Autodesk Inventor part; units mm, degrees
ref_plane "YZ Plane" through (0, 0, 0) normal (1, 0, 0) x (0, 1, 0)
ref_plane "XZ Plane" through (0, 0, 0) normal (0, 1, 0) x (-1, 0, 0)
ref_plane "XY Plane" through (0, 0, 0) normal (0, 0, 1) x (1, 0, 0)
sketch "スケッチ1" plane through (0, 0, 0) normal (0, 0, 1) x (1, 0, 0)
  line L0 (-32.25, 65) -> (32.25, 65)
  line L1 (32.25, 65) -> (32.25, 47.1)
  line L2 (-32.25, -65) -> (-32.25, -47.1)
  line L3 (-32.25, 65) -> (32.25, -65) construction
  line L4 (32.25, 65) -> (-32.25, -65) construction
  line L5 (-32.25, 45) -> (-37.25, 45)
  line L6 (-37.25, 15) -> (-32.25, 15)
  line L7 (-37.25, 15) -> (-37.25, 45)
  line L8 (-32.25, -15) -> (-37.25, -15)
  line L9 (-37.25, -15) -> (-37.25, -45)
  line L10 (-37.25, -45) -> (-32.25, -45)
  arc A0 (-32.25, 45) -> (-32.25, 47.1) centre (-32.25, 46.05) ccw
  arc A1 (-32.25, 12.9) -> (-32.25, 15) centre (-32.25, 13.95) ccw
  arc A2 (-32.25, -15) -> (-32.25, -12.9) centre (-32.25, -13.95) ccw
  arc A3 (-32.25, -47.1) -> (-32.25, -45) centre (-32.25, -46.05) ccw
  line L11 (-32.25, 47.1) -> (-32.25, 65)
  line L12 (-32.25, 12.9) -> (-32.25, 15) construction
  line L13 (-32.25, -12.9) -> (-32.25, 12.9)
  line L14 (-32.25, -47.1) -> (-32.25, -45) construction
  line L15 (0, 65) -> (0, -65) construction
  arc A4 (32.25, -45) -> (32.25, -47.1) centre (32.25, -46.05) ccw
  line L16 (37.25, -45) -> (32.25, -45)
  line L17 (37.25, -15) -> (37.25, -45)
  line L18 (32.25, -15) -> (37.25, -15)
  arc A5 (32.25, -12.9) -> (32.25, -15) centre (32.25, -13.95) ccw
  arc A6 (32.25, 15) -> (32.25, 12.9) centre (32.25, 13.95) ccw
  line L19 (37.25, 15) -> (37.25, 45)
  line L20 (37.25, 15) -> (32.25, 15)
  line L21 (32.25, 45) -> (37.25, 45)
  arc A7 (32.25, 47.1) -> (32.25, 45) centre (32.25, 46.05) ccw
  line L22 (32.25, 47.1) -> (32.25, 45) construction
  line L23 (32.25, 12.9) -> (32.25, -12.9)
  line L24 (32.25, -47.1) -> (32.25, -65)
  line L25 (32.25, -12.9) -> (32.25, -15) construction
  line L26 (-32.25, -15) -> (-32.25, -12.9) construction
  line L27 (-32.25, -45) -> (-32.25, -15)
  line L28 (32.25, -15) -> (32.25, -45)
  line L29 (32.25, -45) -> (32.25, -47.1) construction
  line L30 (-20, -11.25) -> (-15, -11.25) construction
  line L31 (-15, -11.25) -> (-15, -31.25) construction
  line L32 (-15, -31.25) -> (-20, -31.25) construction
  line L33 (-20, -31.25) -> (-20, -11.25) construction
  line L34 (-20, -11.25) -> (-15, -31.25) construction
  line L35 (-15, -11.25) -> (-20, -31.25) construction
  line L36 (-20, 2.5) -> (-15, 2.5) construction
  line L37 (-15, 2.5) -> (-15, -45) construction
  line L38 (-15, -45) -> (-20, -45) construction
  line L39 (-20, -45) -> (-20, 2.5) construction
  line L40 (-20, 2.5) -> (-15, -45) construction
  line L41 (-15, 2.5) -> (-20, -45) construction
  circle A8 centre (-17.5, -36.25) radius 1.55
  line L42 (-20, -21.25) -> (-15, -21.25) construction
  line L43 (-17.5, 2.5) -> (-17.5, -45) construction
  circle A9 centre (-17.5, -6.25) radius 1.55
  circle A10 centre (17.5, -36.25) radius 1.55
  circle A11 centre (17.5, -6.25) radius 1.55
  line L44 (32.25, -65) -> (16.75, -65)
  line L45 (-12.5, -62.5) -> (-12.5, -45)
  line L46 (-12.5, -45) -> (0, -45)
  line L47 (12.5, -62.5) -> (12.5, -45)
  line L48 (12.5, -45) -> (0, -45)
  line L49 (-16.75, -65) -> (-32.25, -65)
  line L50 (16.75, -65) -> (-16.75, -65)
  line L51 (-32.25, 45) -> (-32.25, 47.1) construction
  line L52 (-32.25, 15) -> (-32.25, 45)
  line L53 (32.25, 15) -> (32.25, 12.9) construction
  line L54 (32.25, 45) -> (32.25, 15)
  circle A12 centre (-24.5, 43.5) radius 1.25
  line L55 (-32.25, 0) -> (32.25, 0) construction
  line L56 (-32.25, 46.5) -> (32.25, 46.5) construction
  circle A13 centre (-24.5, -61.5) radius 1.25
  circle A14 centre (24.5, 43.5) radius 1.25
  circle A15 centre (24.5, -61.5) radius 1.25
  circle A16 centre (-17.5, -36.25) radius 3 construction
  line L57 (-12.5, -62.5) -> (12.5, -62.5)
  line L58 (-24.25, 40.5) -> (24.25, 40.5)
  line L59 (24.25, 2.5) -> (-24.25, 2.5)
  line L60 (-24.25, 2.5) -> (-24.25, 40.5)
  line L61 (24.25, 2.5) -> (24.25, 40.5)
  line L62 (-20.05, -29.8151) -> (-18.5651, -31.3) construction
  line L63 (-19.3075, -30.5575) -> (-20.05, -31.3) construction
  arc A17 (-20.05, -29.8151) -> (-18.5651, -31.3) centre (-19.3075, -30.5575) ccw
  line L64 (-20.05, -11.2) -> (-18.5651, -11.2) construction
  line L65 (-14.95, -11.2) -> (-14.95, -12.6849) construction
  line L66 (-14.95, -31.3) -> (-16.4349, -31.3) construction
  line L67 (-20.05, -31.3) -> (-20.05, -29.8151) construction
  line L68 (-20.05, -11.2) -> (-14.95, -31.3) construction
  line L69 (-14.95, -11.2) -> (-20.05, -31.3) construction
  arc A18 (-16.4349, -31.3) -> (-14.95, -29.8151) centre (-15.6925, -30.5575) ccw
  arc A19 (-18.5651, -11.2) -> (-20.05, -12.6849) centre (-19.3075, -11.9425) ccw
  arc A20 (-14.95, -12.6849) -> (-16.4349, -11.2) centre (-15.6925, -11.9425) ccw
  line L70 (-20.05, -29.8151) -> (-20.05, -12.6849)
  line L71 (-18.5651, -31.3) -> (-20.05, -31.3) construction
  line L72 (-16.4349, -31.3) -> (-18.5651, -31.3)
  line L73 (-14.95, -29.8151) -> (-14.95, -31.3) construction
  line L74 (-20.05, -12.6849) -> (-20.05, -11.2) construction
  line L75 (-18.5651, -11.2) -> (-16.4349, -11.2)
  line L76 (-16.4349, -11.2) -> (-14.95, -11.2) construction
  line L77 (-14.95, -12.6849) -> (-14.95, -29.8151)
  arc A21 (18.5651, -31.3) -> (20.05, -29.8151) centre (19.3075, -30.5575) ccw
  arc A22 (14.95, -29.8151) -> (16.4349, -31.3) centre (15.6925, -30.5575) ccw
  arc A23 (16.4349, -11.2) -> (14.95, -12.6849) centre (15.6925, -11.9425) ccw
  arc A24 (20.05, -12.6849) -> (18.5651, -11.2) centre (19.3075, -11.9425) ccw
  line L78 (20.05, -29.8151) -> (20.05, -12.6849)
  line L79 (16.4349, -31.3) -> (18.5651, -31.3)
  line L80 (18.5651, -11.2) -> (16.4349, -11.2)
  line L81 (14.95, -12.6849) -> (14.95, -29.8151)
  line L82 (-32.25, -65) -> (-32.25, -70)
  line L83 (-32.25, -70) -> (32.25, -70)
  line L84 (32.25, -70) -> (32.25, -65)
  point P0 (0, 0)
  point P1 (0, 0)
  point P2 (0, 0)
  point P3 (28, 15)
  point P4 (28, 45)
  point P5 (-17.5, -21.25)
  point P6 (28, 45)
  point P7 (28, 15)
  dimension "d0" = 64.5
  dimension "d1" = 130
  dimension "d2" = 20
  dimension "d3" = 30
  dimension "d4" = 30
  dimension "d5" = 30
  dimension "d6" = 1.05
  dimension "d7" = 1.05
  dimension "d8" = 1.05
  dimension "d9" = 1.05
  dimension "d10" = 5
  dimension "d23" = 15
  dimension "d24" = 5
  dimension "d25" = 20
  dimension "d28" = 3.1
  dimension "d72" = 47.5
  dimension "d103" = 12.25
  dimension "d109" = 71.25
  dimension "d111" = 20
  dimension "d113" = 7.75
  dimension "d114" = 2.5
  dimension "d115" = 18.5
  dimension "d116" = 3
  dimension "d117" = 2.5
  dimension "d118" = 7.75
  dimension "d119" = 3.5
  dimension "d120" = 25
  dimension "d121" = 6
  dimension "d124" = 2.5
  dimension "d126" = 8
  dimension "d128" = 6
  dimension "d130" = 1.05
  dimension "d131" = 0.05
  dimension "d132" = 0.05
  dimension "d133" = 5
  dimension "d157" = 25
  dimension "d158" = 30
extrude "押し出し1" add sketch "スケッチ1" along normal blind 2.5 contours L0 L1 A7 L54 A6 L23 A5 L28 A4 L24 L44 L50 L49 L2 A3 L27 A2 L13 A1 L52 A0 L11 | L52 L6 L7 L5 | L21 L19 L20 L54 | L27 L10 L9 L8 | L18 L17 L16 L28
extrude "押し出し2" add sketch "スケッチ1" along normal blind 5 contours L0 L1 A7 L54 A6 L23 A5 L28 A4 L24 L44 L50 L49 L2 A3 L27 A2 L13 A1 L52 A0 L11
fillet "フィレット1" radius 1 7 edges at (-12.5, -45, 2.5) (-12.5, -62.5, 2.5) (12.5, -62.5, 2.5) (-24.25, 40.5, 2.5) (24.25, 40.5, 2.5) (24.25, 2.5, 2.5) (-24.25, 2.5, 2.5)
sketch "スケッチ7" plane through (32.25, -70, 0) normal (1, 0, 0) x (0, 0, -1)
  line L0 (0, 55) -> (-2.5, 55)
  line L1 (0, 57.1) -> (0, 82.9)
  line L2 (0, 5) -> (0, 22.9)
  point P0 (0, 70)
  point P1 (-2.5, 15)
  point P2 (-2.5, 65)
  point P3 (0, 25)
  dimension "d136" = 10
  dimension "d137" = 10
  dimension "d138" = 2.5
  dimension "d139" = 2.5
hole "穴6" at (32.25, -55, 2.5) at (32.25, -5, 2.5) direction (-1, 0, 0) diameter 2.459 depth 4
sketch "スケッチ8" plane through (-32.25, -70, 0) normal (-1, 0, 0) x (0, 0, 1)
  circle A0 centre (2.5, 15) radius 1.2295
  circle A1 centre (2.5, 65) radius 1.2295
  point P0 (0, 70)
  point P1 (2.5, 15)
  point P2 (2.5, 65)
hole "穴7" at (-32.25, -5, 2.5) at (-32.25, -55, 2.5) direction (1, 0, 0) diameter 2.459 depth 4
chamfer "面取り2" distance 0.5 angle 45 8 edges at (-37.25, -45, 1.25) (-37.25, -15, 1.25) (-37.25, 15, 1.25) (-37.25, 45, 1.25) (37.25, 15, 1.25) (37.25, 45, 1.25) (37.25, -15, 1.25) (37.25, -45, 1.25)
equation "\"d2\" = -0.5 * d4 + 0.5 * d1 - d3"
equation "\"d5\" = d3"
equation "\"d7\" = d6"
equation "\"d8\" = d7"
equation "\"d9\" = d8"
properties part number "Cockpit_upper_bottom_frame" material "アセタール樹脂、黒"
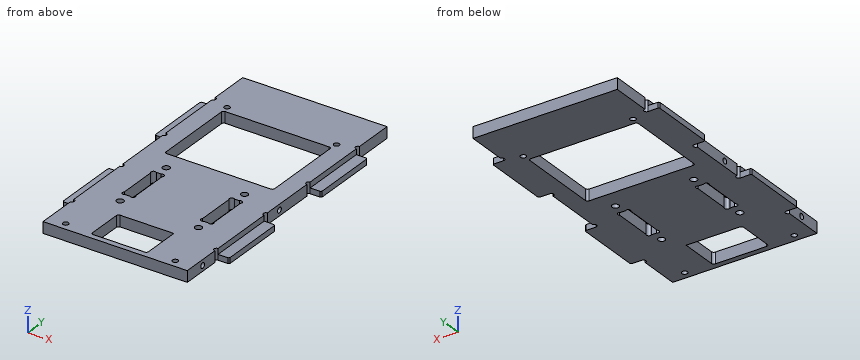
Work out the finished part from the listing and answer in its coordinate system (mm). Give positions to 0.01 mm unless a question says otherwise; leave off trailing zeros. Write each loop counter-clockwise with the first axis right and the second up, starting at its lowest first coordinate (ties: lowest second). Pieces come first, ordered by that corner, then holes. Notation, with made-up numbers: M 53,42 L 111,42 A27 ccw 111,71 Z; hole C 76.5,66 d9. An arc over 180 degrees is marked long. Answer as CSV lines item,"result".
Q1. A cutting plane is placed at B-B on y = 36.5. Write down the section's boundary in (x, z).
A:
outline,"M -37.25,0 L -24.25,0 L -24.25,5 L -32.25,5 L -32.25,2.5 L -37.25,2.5 Z; M 24.25,0 L 37.25,0 L 37.25,2.5 L 32.25,2.5 L 32.25,5 L 24.25,5 Z"
Q2. Given P1, Ø2.5, axis at x = 34, y = -35, coming from the +Z side; P2, Ø2, axis at y = -5, z = 2.5, coming from the -X side; P3, Ø1.5, axis at x = 27, y = 16, coming from the -Z side; P4, Ø0.8, axis at x = -35, z = 1, coming from the +Y side, each flat-ended and moving along its own axis, determine where each tip first touches the part or whether it passes through.
A:
P1,"stops at z = 2.5"
P2,"stops at x = -28.25"
P3,"stops at z = 0"
P4,"stops at y = 45"
Q3. A cutting plane is placed at D-D on y = 6. Write down the section's boundary in (x, z).
A:
outline,"M -32.25,0 L -24.25,0 L -24.25,5 L -32.25,5 Z; M 24.25,0 L 32.25,0 L 32.25,5 L 24.25,5 Z"
Q4. A cutting plane is placed at A-A on y = -36.25. Write down the section's boundary in (x, z).
A:
outline,"M -37.25,0 L -19.05,0 L -19.05,5 L -32.25,5 L -32.25,2.5 L -37.25,2.5 Z; M -15.95,0 L 15.95,0 L 15.95,5 L -15.95,5 Z; M 19.05,0 L 37.25,0 L 37.25,2.5 L 32.25,2.5 L 32.25,5 L 19.05,5 Z"
Q5. A cutting plane is placed at C-C on x = 5. Write down the section's boundary in (y, z).
A:
outline,"M -65,0 L -62.5,0 L -62.5,5 L -65,5 Z; M -45,0 L 2.5,0 L 2.5,5 L -45,5 Z; M 40.5,0 L 65,0 L 65,5 L 40.5,5 Z"
Q6. Find the intervals of material crossed by probe 1 along X at (y, z) = (-27.5, 4.2); probe 2 along Y at (x, z) = (5, 0.75); probe 3 along Y at (x, z) = (-24.5, 3), in increasing order. Write a range as [from, to].
A:
probe 1,"x = [-32.25, -20.05], [-14.95, 14.95], [20.05, 32.25]"
probe 2,"y = [-65, -62.5], [-45, 2.5], [40.5, 65]"
probe 3,"y = [-65, -62.75], [-60.25, 42.25], [44.75, 65]"
